Read the model definition and answer for the solid it produces. Units are mm, in the model's axes. Face numbers are marked on the shaded views. A direction names the side the tool comes from. Coordinates: 2 decimals unless noted, no trailing zeros. Order: outer loops, then holes, each group sorted by start corner. A loop starts at its lowest first (then second) coordinate and runs counter-clockwise, first axis right, second up.
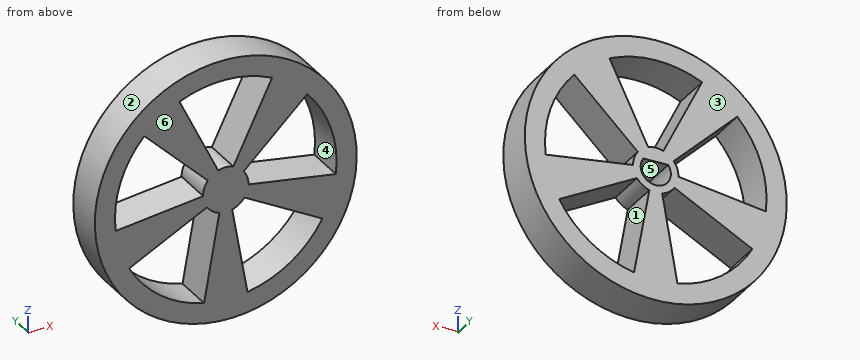
```python
from build123d import *

# Parameters (mm, degrees)
SKETCH1_R           = 13
BOSS_EXTRUDE1_DEPTH = 4
SKETCH1_4_R         = 1.5
BOSS_EXTRUDE2_DEPTH = 0.5


with BuildPart() as part:
    # Sketch1 → Boss-Extrude1 (new body)
    with BuildSketch(Plane(origin=(0, 0, 0), x_dir=(1, 0, 0), z_dir=(0, 1, 0))):
        with Locations(Location((0, 0, 0), (0, 0, 270))):
            Circle(SKETCH1_R)
        with BuildLine():
            ThreePointArc((-2.249114933, 0.063103228), (-2.139877162, -0.695288237), (-1.782481056, -1.373048173))
            Line((-1.782481056, -1.373048173), (-8.084716138, -7.459045848))
            ThreePointArc((-8.084716138, -7.459045848), (-10.461621679, -3.399186938), (-10.924989896, 1.282417938))
            Line((-10.924989896, 1.282417938), (-2.249114933, 0.063103228))
        make_face(mode=Mode.SUBTRACT)
        with BuildLine():
            ThreePointArc((-0.755029473, -2.119535443), (0, -2.25), (0.755029473, -2.119535443))
            Line((0.755029473, -2.119535443), (4.595659477, -9.993993895))
            ThreePointArc((4.595659477, -9.993993895), (0, -11), (-4.595659477, -9.993993895))
            Line((-4.595659477, -9.993993895), (-0.755029473, -2.119535443))
        make_face(mode=Mode.SUBTRACT)
        with BuildLine():
            ThreePointArc((1.782481056, -1.373048173), (2.139877162, -0.695288237), (2.249114933, 0.063103228))
            Line((2.249114933, 0.063103228), (10.924989896, 1.282417938))
            ThreePointArc((10.924989896, 1.282417938), (10.461621679, -3.399186938), (8.084716138, -7.459045848))
            Line((8.084716138, -7.459045848), (1.782481056, -1.373048173))
        make_face(mode=Mode.SUBTRACT)
        with BuildLine():
            ThreePointArc((-0.635, 2.158535383), (-1.322516818, 1.820288237), (-1.85666335, 1.270945004))
            Line((-1.85666335, 1.270945004), (-9.59228884, 5.384050037))
            ThreePointArc((-9.59228884, 5.384050037), (-6.465637775, 8.899186938), (-2.156355605, 10.786571768))
            Line((-2.156355605, 10.786571768), (-0.635, 2.158535383))
        make_face(mode=Mode.SUBTRACT)
        with BuildLine():
            Line((1.235920709, -0.85), (-1.235920709, -0.85))
            ThreePointArc((-1.235920709, -0.85), (0, 1.5), (1.235920709, -0.85))
        make_face(mode=Mode.SUBTRACT)
        with BuildLine():
            Line((0.635, 2.158535383), (2.156355605, 10.786571768))
            ThreePointArc((2.156355605, 10.786571768), (6.465637775, 8.899186938), (9.59228884, 5.384050037))
            Line((9.59228884, 5.384050037), (1.85666335, 1.270945004))
            ThreePointArc((1.85666335, 1.270945004), (1.322516818, 1.820288237), (0.635, 2.158535383))
        make_face(mode=Mode.SUBTRACT)
    extrude(amount=BOSS_EXTRUDE1_DEPTH)

    # Sketch1_4 → Boss-Extrude2 (add)
    with BuildSketch(Plane(origin=(0, 0, 0), x_dir=(1, 0, 0), z_dir=(0, 1, 0))):
        Circle(SKETCH1_4_R)
    extrude(amount=BOSS_EXTRUDE2_DEPTH)


solid = part.part
```
1) A cutting plane is placed at B-B, the plane y = 3.55. Determine the outline of the cut face in (x, z) (3 decimals), and give its area (3 significant figures).
A:
outline: circle Ø26 at (0, 0); hole (-10.925, -1.282) - (-2.249, -0.063) arc R2.25 cw to (-1.782, 1.373) - (-8.085, 7.459) arc R11 ccw to start; hole (-9.592, -5.384) arc R11 ccw to (-2.156, -10.787) - (-0.635, -2.159) arc R2.25 cw to (-1.857, -1.271) - close; hole (-4.596, 9.994) - (-0.755, 2.12) arc R2.25 cw to (0.755, 2.12) - (4.596, 9.994) arc R11 ccw to start; hole (-1.236, 0.85) arc R1.5 ccw (long way) to (1.236, 0.85) - close; hole (0.635, -2.159) - (2.156, -10.787) arc R11 ccw to (9.592, -5.384) - (1.857, -1.271) arc R2.25 cw to start; hole (1.782, 1.373) arc R2.25 cw to (2.249, -0.063) - (10.925, -1.282) arc R11 ccw to (8.085, 7.459) - close
area: 284 mm2
2) Straight lines are drawn through the part: line 1 (X direction, y = 2.9, z = 0); line 2 (X direction, y = 3.25, z = 6.75); line 3 (Z direction, x = 5.25, y = 3.6). For each, find the intervals that lie inside material, in ascending order.
A:
line 1: x = -13 to -11, -2.25 to -1.5, 1.5 to 2.25, 11 to 13
line 2: x = -11.11 to -8.69, -7.35 to -3.01, 3.01 to 7.35, 8.69 to 11.11
line 3: z = -11.89 to -9.67, -3.08 to -0.48, 4.72 to 11.89
3) A cutting plane is placed at D-D, the plane z = -2.5. Determine the outline of the cut face in (x, y), and give its area (3 significant figures).
A:
outline: (-12.76, 0) - (-4.17, 0) - (-4.17, 4) - (-12.76, 4) - close; (-0.7, 0) - (0.7, 0) - (0.7, 4) - (-0.7, 4) - close; (4.17, 0) - (12.76, 0) - (12.76, 4) - (4.17, 4) - close
area: 74.3 mm2
4) A cutting plane is placed at A-A, the plane x = 0. Determine the outline of the cut face in (y, z), and give its area (3 significant figures).
A:
outline: (0, -13) - (4, -13) - (4, -1.5) - (0.5, -1.5) - (0.5, 0.85) - (4, 0.85) - (4, 2.25) - (0, 2.25) - close; (0, 11) - (4, 11) - (4, 13) - (0, 13) - close
area: 60.8 mm2
5) A cutting plane is placed at C-C, the plane x = 6.5. Determine the outline of the cut face in (y, z).
A:
outline: (0, -11.26) - (4, -11.26) - (4, -8.87) - (0, -8.87) - close; (0, -3.74) - (4, -3.74) - (4, -0.66) - (0, -0.66) - close; (0, 5.93) - (4, 5.93) - (4, 11.26) - (0, 11.26) - close
6) Which of the six approach directions +Z, -Z, +X, -X, +Y, -Y give full straight-line access (tool end or side, diameter ignored) to the marked faces 4, 5 and 6?
A:
face 4: +Y, -Y
face 5: +Y
face 6: +Z, -Z, +X, -X, -Y
7) A flat-ended cylindrical pin translates along its axis: pin 1 Ø1 at (x, y) = (5.5, 1) entering from +Z. Find the tip coordinate at first contact, or state that the pin passes through.
A:
pin 1: stops at z = 12
8) Determine the mould class of the marked faces 1, 2 and 3 for opening direction X: pulls with the +X half, pulls with the -X half, needs draft (parallel to the pull), parting line crosses it, or undercut.
A:
face 1: undercut
face 2: parting line crosses it
face 3: needs draft
